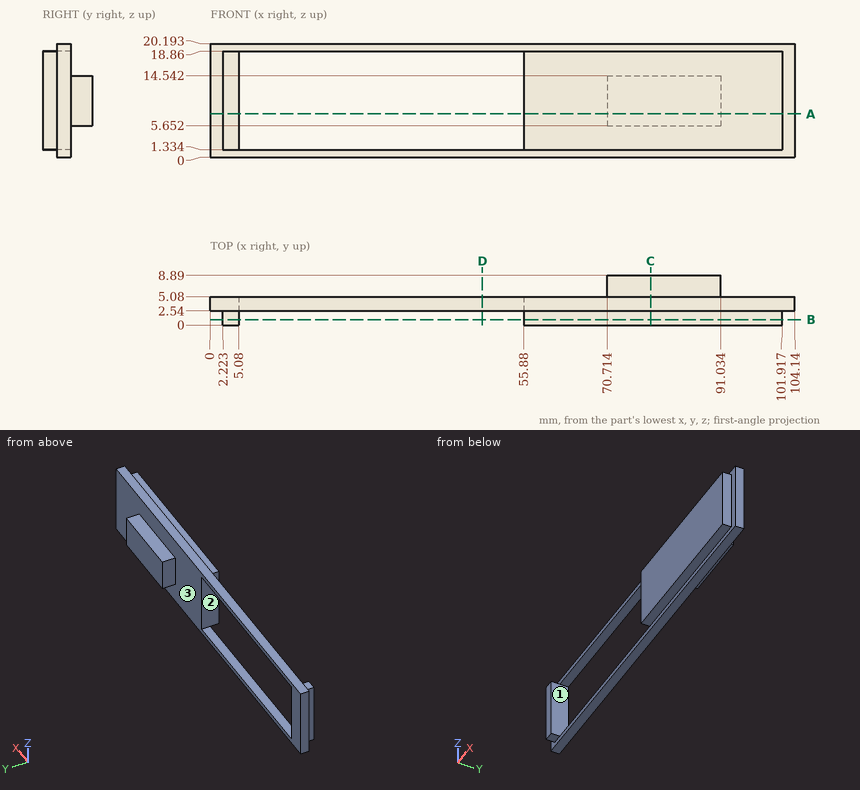
Verification items for this drawing (mm, ordinates from the low corner). Give positions to 0.01 mm unless a question says otherwise; leave off trailing zeros. Write each loop counter-clockwise with the first axis right and the second up, starting at its lowest first coordinate (ties: lowest second). Pieces come first, ordered by that corner, then holes. Notation, with made-up numbers: (50, -34) - (79, -34) arc R20 ccw to (79, -9) - close; hole circle Ø11 at (72, 9). An arc over 180 degrees is marked (long way). Answer as a JSON object with one key per item and string values. Group by question number.
1) Sectioned sample at C-C (x = 78.5). Record the cut outline in (y, z), then the cut area to 3 significant figures.
2) Sectioned sample at D-D (x = 48.5). Record the cut outline in (y, z).
3) Release check for a two-part mould opening along X. For the marked faces 1, 2 and 3 record: pulls with the +X half, pulls with the -X half, needs draft (parallel to the pull), parting line crosses it, or undercut.
4) Sectioned sample at A-A (z = 7.75). Record the cut outline in (x, y), then the cut area to 3 significant figures.
5) Thickness scan on probe 1 along X at (y, z) = (4.75, 15.25); probe 2 along Z at (x, y) = (43, 3.5); probe 3 along X at (y, z) = (2.25, 2.5). Record the ranges inside material, lowest first. Write a range as from..to.
6) Depth check by flat-ended pin: P1, Ø1, axis at y = 6.5, z = 9.5, coming from the +X side; P2, Ø0.8, axis at y = 0.5, z = 7, coming from the +X side; P3, Ø3, axis at y = 1, z = 13, coming from the -X side. Enter the tip coordinate at first touch or a pass-through.
7) Sectioned sample at B-B (y = 1). Record the cut outline in (x, z), then the cut area to 3 significant figures.
Geometry results:
{
 "1": {"outline": "(0, 1.33) - (2.54, 1.33) - (2.54, 0) - (5.08, 0) - (5.08, 5.65) - (8.89, 5.65) - (8.89, 14.54) - (5.08, 14.54) - (5.08, 20.19) - (2.54, 20.19) - (2.54, 18.86) - (0, 18.86) - close", "area": "130 mm^2"},
 "2": {"outline": "(2.54, 0) - (5.08, 0) - (5.08, 1.33) - (2.54, 1.33) - close; (2.54, 18.86) - (5.08, 18.86) - (5.08, 20.19) - (2.54, 20.19) - close"},
 "3": {"face 1": "undercut", "face 2": "undercut", "face 3": "needs draft"},
 "4": {"outline": "(0, 2.54) - (2.22, 2.54) - (2.22, 0) - (5.08, 0) - (5.08, 5.08) - (0, 5.08) - close; (55.88, 0) - (101.92, 0) - (101.92, 2.54) - (104.14, 2.54) - (104.14, 5.08) - (91.03, 5.08) - (91.03, 8.89) - (70.71, 8.89) - (70.71, 5.08) - (55.88, 5.08) - close", "area": "337 mm^2"},
 "5": {"probe 1": "x = 0..5.08, 55.88..104.14", "probe 2": "z = 0..1.33, 18.86..20.19", "probe 3": "x = 2.22..5.08, 55.88..101.92"},
 "6": {"P1": "stops at x = 91.03", "P2": "stops at x = 101.92", "P3": "stops at x = 2.22"},
 "7": {"outline": "(2.22, 1.33) - (5.08, 1.33) - (5.08, 18.86) - (2.22, 18.86) - close; (55.88, 1.33) - (101.92, 1.33) - (101.92, 18.86) - (55.88, 18.86) - close", "area": "857 mm^2"}
}
